from build123d import *

# Parameters (mm, degrees)
SKETCH1_R           = 3.175
BOSS_EXTRUDE1_DEPTH = 6.35


with BuildPart() as part:
    # Sketch1 → Boss-Extrude1 (new body)
    with BuildSketch(Plane.XY):
        Polygon((0, 13.506188545), (0, 178.506188545), (50.8, 178.506188545), (50.8, 13.506188545), (63.5, 13.506188545), (63.5, -11.893811455), (-12.7, -11.893811455), (-12.7, 13.506188545), align=None)
        with Locations((6.35, -2.604847725)):
            Circle(SKETCH1_R, mode=Mode.SUBTRACT)
        with Locations((44.45, -2.604847725)):
            Circle(SKETCH1_R, mode=Mode.SUBTRACT)
        with Locations((25.4, 165.806188545)):
            Circle(SKETCH1_R, mode=Mode.SUBTRACT)
        with Locations((25.4, 140.406188545)):
            Circle(SKETCH1_R, mode=Mode.SUBTRACT)
        with Locations((25.4, 115.006188545)):
            Circle(SKETCH1_R, mode=Mode.SUBTRACT)
        with Locations((25.4, 89.606188545)):
            Circle(SKETCH1_R, mode=Mode.SUBTRACT)
        with Locations((25.4, 64.206188545)):
            Circle(SKETCH1_R, mode=Mode.SUBTRACT)
    extrude(amount=BOSS_EXTRUDE1_DEPTH)


solid = part.part
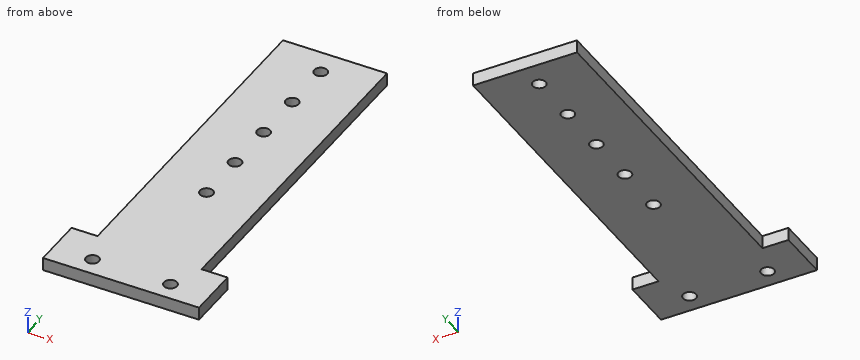
Geometry check sheet. Reference: the model listing, model coordinates, mm. Coordinates: 2 decimals unless noted, no trailing zeros. Loops run counter-clockwise (first coordinate to the right, second up) from the corner with the lowest first, then second, coordinate; pieces in that order, holes last. Notation, with made-up numbers: (51.25, 34.5) - (57.25, 34.5) arc R21 ccw to (57.25, 65.5) - close; hole circle Ø11 at (0.5, 42). An arc over 180 degrees is marked (long way). Use one line per item in the form item = value. Start each with the question number.
Item 1: Thickness scan on probe 1 along Y at (x, z) = (25.4, 4.25); probe 2 along Y at (x, z) = (24.5, 1.25); probe 3 along X at (y, z) = (90, 1). Record the ranges inside material, lowest first.
Item 2: Section check C-C, the plane z = 5.25. Enter the section's corners in (x, y) (3 decimals), and give its area (3 significant figures).
Item 3: Section check B-B, the plane x = 44.45. Enter the section's corners in (y, z), and give its area (3 significant figures).
Item 4: Section check D-D, the plane y = 49.5. Enter the section's corners in (x, z), and give its area (3 significant figures).
Item 5: Section check A-A, the plane x = 25.4. Enter the section's corners in (y, z), and give its area (3 significant figures).
Item 6: Gauge pin test, flat ends, axial feed: pin 1 (7.5 mm diameter, centred on x = 25.4, y = 115.01, fed in from +Z); pin 2 (1.9 mm diameter, centred on y = 114, z = 2.5, fed in from +X); pin 3 (3 mm diameter, centred on x = 59.5, z = 3, fed in from +Y); pin 4 (1.9 mm diameter, centred on y = 65, z = 4, fed in from -X). Record the tip position at first contact, or that the pin passes through.
Computed:
q1.probe_1 = -11.89 to 61.03, 67.38 to 86.43, 92.78 to 111.83, 118.18 to 137.23, 143.58 to 162.63, 168.98 to 178.51
q1.probe_2 = -11.89 to 61.16, 67.25 to 86.56, 92.65 to 111.96, 118.05 to 137.36, 143.45 to 162.76, 168.85 to 178.51
q1.probe_3 = 0 to 22.25, 28.55 to 50.8
q2.outline = (-12.7, -11.894) - (63.5, -11.894) - (63.5, 13.506) - (50.8, 13.506) - (50.8, 178.506) - (0, 178.506) - (0, 13.506) - (-12.7, 13.506) - close; hole circle Ø6.35 at (6.35, -2.605); hole circle Ø6.35 at (25.4, 64.206); hole circle Ø6.35 at (25.4, 89.606); hole circle Ø6.35 at (25.4, 115.006); hole circle Ø6.35 at (25.4, 140.406); hole circle Ø6.35 at (25.4, 165.806); hole circle Ø6.35 at (44.45, -2.605)
q2.area = 10,100 mm2
q3.outline = (-11.89, 0) - (-5.78, 0) - (-5.78, 6.35) - (-11.89, 6.35) - close; (0.57, 0) - (178.51, 0) - (178.51, 6.35) - (0.57, 6.35) - close
q3.area = 1,170 mm2
q4.outline = (0, 0) - (50.8, 0) - (50.8, 6.35) - (0, 6.35) - close
q4.area = 323 mm2
q5.outline = (-11.89, 0) - (61.03, 0) - (61.03, 6.35) - (-11.89, 6.35) - close; (67.38, 0) - (86.43, 0) - (86.43, 6.35) - (67.38, 6.35) - close; (92.78, 0) - (111.83, 0) - (111.83, 6.35) - (92.78, 6.35) - close; (118.18, 0) - (137.23, 0) - (137.23, 6.35) - (118.18, 6.35) - close; (143.58, 0) - (162.63, 0) - (162.63, 6.35) - (143.58, 6.35) - close; (168.98, 0) - (178.51, 0) - (178.51, 6.35) - (168.98, 6.35) - close
q5.area = 1,010 mm2
q6.pin_1 = 6.35
q6.pin_2 = 50.8
q6.pin_3 = 13.51
q6.pin_4 = 0
